Geometry: final body of the model. Coordinates: model frame, mm. Face numbers are marked on the shaded views. Give positions to 0.01 mm unless a question says otherwise; leave off trailing zeros. Write each loop counter-clockwise with the first axis right and the second up, starting at its lowest first coordinate (ties: lowest second). Pieces come first, ordered by that corner, then holes. Notation, with made-up numbers: (68.5, 43.5) -> (111.5, 43.5) arc R31 ccw to (111.5, 77.5) -> close; hole circle Ø11 at (68, -32). An arc over 180 degrees is marked (long way). Answer as a JSON object with one key per item and string values.
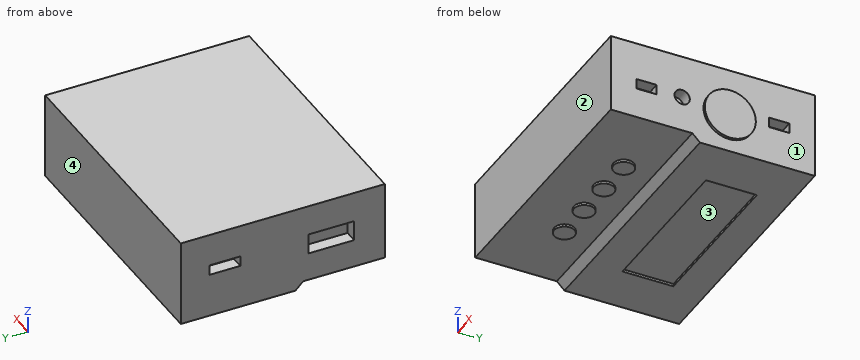
from build123d import *

# Parameters (mm, degrees)
ESQUISSE1_W             = 103
ESQUISSE1_H             = 80
BOSS_EXTRU_1_DEPTH      = 34
ENL_V_MAT_EXTRU_2_DEPTH = 224
ESQUISSE3_W             = 63.460243042
ESQUISSE3_H             = 20
ENL_V_MAT_EXTRU_3_DEPTH = 1
ESQUISSE4_R             = 4
BOSS_EXTRU_2_DEPTH      = 1
ESQUISSE5_R             = 3
ESQUISSE5_W             = 4
ESQUISSE5_H             = 8
ENL_V_MAT_EXTRU_4_DEPTH = 5
ESQUISSE6_R             = 10
BOSS_EXTRU_3_DEPTH      = 1
ESQUISSE7_W             = 8
ESQUISSE7_H             = 18
ESQUISSE7_W_2           = 4
ESQUISSE7_H_2           = 12
ENL_V_MAT_EXTRU_5_DEPTH = 5


with BuildPart() as part:
    # Esquisse1 → Boss.-Extru.1 (new body)
    with BuildSketch(Plane.XY):
        Rectangle(ESQUISSE1_W, ESQUISSE1_H)
    extrude(amount=BOSS_EXTRU_1_DEPTH)

    # Esquisse2 → Enlèv. mat.-Extru.2 (cut)
    with BuildSketch(Plane.ZY.offset(51.5)):
        Polygon((3, -8), (0, -5), (0, -40), (3, -40), (3, -37), align=None)
    extrude(amount=-ENL_V_MAT_EXTRU_2_DEPTH, mode=Mode.SUBTRACT)

    # Esquisse3 → Enlèv. mat.-Extru.3 (cut)
    with BuildSketch(Plane(origin=(0, 0, 0), x_dir=(-1, 0, 0), z_dir=(0, 0, -1))):
        with Locations((0, 17.5)):
            Rectangle(ESQUISSE3_W, ESQUISSE3_H)
    extrude(amount=-ENL_V_MAT_EXTRU_3_DEPTH, mode=Mode.SUBTRACT)

    # Esquisse4 → Boss.-Extru.2 (add)
    with BuildSketch(Plane(origin=(0, 0, 3), x_dir=(-1, 0, 0), z_dir=(0, 0, -1))):
        with Locations((-7.5, -20)):
            Circle(ESQUISSE4_R)
        with Locations((-22.5, -20)):
            Circle(ESQUISSE4_R)
        with Locations((7.5, -20)):
            Circle(ESQUISSE4_R)
        with Locations((22.5, -20)):
            Circle(ESQUISSE4_R)
    extrude(amount=BOSS_EXTRU_2_DEPTH)

    # Esquisse5 → Enlèv. mat.-Extru.4 (cut)
    with BuildSketch(Plane(origin=(51.5, 0, 0), x_dir=(0, 0, -1), z_dir=(1, 0, 0))):
        with Locations((-17, -12)):
            Circle(ESQUISSE5_R)
        with Locations((-17, 26)):
            Rectangle(ESQUISSE5_W, ESQUISSE5_H)
        with Locations((-17, -26)):
            Rectangle(ESQUISSE5_W, ESQUISSE5_H)
    extrude(amount=-ENL_V_MAT_EXTRU_4_DEPTH, mode=Mode.SUBTRACT)

    # Esquisse6 → Boss.-Extru.3 (add)
    with BuildSketch(Plane(origin=(51.5, 0, 0), x_dir=(0, 0, -1), z_dir=(1, 0, 0))):
        with Locations((-15, 6.367248466)):
            Circle(ESQUISSE6_R)
    extrude(amount=BOSS_EXTRU_3_DEPTH)

    # Esquisse7 → Enlèv. mat.-Extru.5 (cut)
    with BuildSketch(Plane.ZY.offset(51.5)):
        with Locations((18.106114865, -18.992792822)):
            Rectangle(ESQUISSE7_W, ESQUISSE7_H)
        with Locations((19.212725932, 22.654616942)):
            Rectangle(ESQUISSE7_W_2, ESQUISSE7_H_2)
    extrude(amount=-ENL_V_MAT_EXTRU_5_DEPTH, mode=Mode.SUBTRACT)


solid = part.part
Q1. Cut plane A-A (y = -12). Return the cut outline in (x, z), and give its area (3 significant figures).
Values:
{"outline": "(-51.5, 3) -> (51.5, 3) -> (51.5, 14) -> (46.5, 14) -> (46.5, 20) -> (51.5, 20) -> (51.5, 34) -> (-51.5, 34) -> (-51.5, 22.11) -> (-46.5, 22.11) -> (-46.5, 14.11) -> (-51.5, 14.11) -> close", "area": "3,120 mm²"}
Q2. Cut plane D-D (x = 30). Return the cut outline in (y, z).
Values:
{"outline": "(-40, 3) -> (-8, 3) -> (-5, 0) -> (7.5, 0) -> (7.5, 1) -> (27.5, 1) -> (27.5, 0) -> (40, 0) -> (40, 34) -> (-40, 34) -> close"}
Q3. Cut plane C-C (y = -20). Return the cut outline in (x, z), and give its area (4 significant figures).
Values:
{"outline": "(-51.5, 3) -> (-26.5, 3) -> (-26.5, 2) -> (-18.5, 2) -> (-18.5, 3) -> (-11.5, 3) -> (-11.5, 2) -> (-3.5, 2) -> (-3.5, 3) -> (3.5, 3) -> (3.5, 2) -> (11.5, 2) -> (11.5, 3) -> (18.5, 3) -> (18.5, 2) -> (26.5, 2) -> (26.5, 3) -> (51.5, 3) -> (51.5, 34) -> (-51.5, 34) -> (-51.5, 22.11) -> (-46.5, 22.11) -> (-46.5, 14.11) -> (-51.5, 14.11) -> close", "area": "3,185 mm²"}
Q4. Mould query, pull axis Y, two halves, no side actions, for the marked faces 1, 2, 3 and 4. Classes: pulls with the +Y half, pulls with the -Y half, needs draft (parallel to the pull), parting line crosses it, or undercut.
Values:
{"face 1": "needs draft", "face 2": "pulls with the -Y half", "face 3": "undercut", "face 4": "pulls with the +Y half"}
Q5. Cut plane B-B (x = -7.5). Return the cut outline in (y, z).
Values:
{"outline": "(-40, 3) -> (-24, 3) -> (-24, 2) -> (-16, 2) -> (-16, 3) -> (-8, 3) -> (-5, 0) -> (7.5, 0) -> (7.5, 1) -> (27.5, 1) -> (27.5, 0) -> (40, 0) -> (40, 34) -> (-40, 34) -> close"}
Q6. Material intervals for L1, parallel to Y at x = 48.8, z = 17; L2, parallel to Z at x = 3, y = -13; L3, parallel to X at y = -23, z = 16.5, sorted ascending. Write a range as from..to.
Values:
{"L1": "-40..-30, -22..-15, -9..22, 30..40", "L2": "3..34", "L3": "-46.5..46.5"}
Q7. First-contact query: P1, Ø9, axis at x = 9.5, y = -19.5, coming from the -Z side; P2, Ø5.5, axis at x = -49.5, y = -22, coming from the -Z side; P3, Ø4.5, axis at y = -26.5, z = 16.5, coming from the +X side. Flat tips, straight axial feed; report the tip coordinate or a pass-through.
Values:
{"P1": "z = 2", "P2": "z = 3", "P3": "x = 51.5"}
